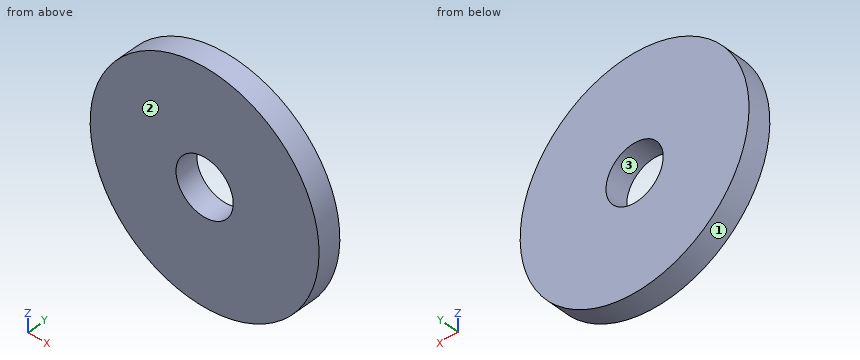
```python
from build123d import *

# Parameters (mm, degrees)
SKETCH1_R           = 12.5
SKETCH1_R_2         = 2.125
BOSS_EXTRUDE1_DEPTH = 2
SKETCH2_R           = 2.5
CUT_EXTRUDE1_DEPTH  = 10
CUT_EXTRUDE2_START  = -10
SKETCH3_R           = 12.5
SKETCH3_R_2         = 10
CUT_EXTRUDE2_DEPTH  = 10


with BuildPart() as part:
    # Sketch1 → Boss-Extrude1 (new body)
    with BuildSketch(Plane(origin=(0, 0, 0), x_dir=(1, 0, 0), z_dir=(0, 1, 0))):
        with Locations(Location((0, 0, 0), (0, 0, 270))):
            Circle(SKETCH1_R)
        with Locations(Location((0, 0, 0), (0, 0, 270))):
            Circle(SKETCH1_R_2, mode=Mode.SUBTRACT)
    extrude(amount=BOSS_EXTRUDE1_DEPTH)

    # Sketch2 → Cut-Extrude1 (cut)
    with BuildSketch(Plane(origin=(0, 2, 0), x_dir=(1, 0, 0), z_dir=(0, 1, 0))):
        with Locations(Location((0, 0, 0), (0, 0, 270))):
            Circle(SKETCH2_R)
    extrude(amount=-CUT_EXTRUDE1_DEPTH, mode=Mode.SUBTRACT)

    # Sketch3 → Cut-Extrude2 (cut)
    with BuildSketch(Plane(origin=(0, 2, 0), x_dir=(1, 0, 0), z_dir=(0, 1, 0)).offset(CUT_EXTRUDE2_START)):
        Circle(SKETCH3_R)
        with Locations(Location((0, 0, 0), (0, 0, 270))):
            Circle(SKETCH3_R_2, mode=Mode.SUBTRACT)
    extrude(amount=CUT_EXTRUDE2_DEPTH, mode=Mode.SUBTRACT)


solid = part.part
```
Verification items for the finished model (mm, model axes). Face numbers are marked on the shaded views. Give positions to 0.01 mm unless a question says otherwise; leave off trailing zeros. Order: outer loops, then holes, each group sorted by start corner. A loop starts at its lowest first (then second) coordinate and runs counter-clockwise, first axis right, second up. Notation, with made-up numbers: M 11.5,82.5 L 48.5,82.5 A3 ccw 48.5,87.5 Z; hole C -21,79.5 d1. An arc over 180 degrees is marked long. Return JSON: item names as keys, results as strings. Group by question number.
1) Scan lines: line 1 (X direction, y = 1.25, z = 0); line 2 (Z direction, x = -1.5, y = 1.6); line 3 (Z direction, x = 0.5, y = 0.25). Record each from-to range of solid material in increasing order.
2) Mould release check, pull along X, two halves, no side actions. Record for the marked faces 1, 2 and 3: pulls with the +X half, pulls with the -X half, needs draft (parallel to the pull), parting line crosses it, or undercut.
3) Section check C-C on y = 0.25. Record the cut outline in (x, z), and give its area (3 significant figures).
4) Section check A-A on z = 0. Record the cut outline in (x, y), and give its area (3 significant figures).
5) Section check D-D on z = 6.75. Record the cut outline in (x, y), and give its area (3 significant figures).
6) Section check B-B on x = 0. Record the cut outline in (y, z).
7) Go/stop test with flat-tipped pins: pin 1 Ø1 at (y, z) = (1, 1.5) entering from -X; pin 2 Ø4 at (x, z) = (0, 0) entering from +Y. Record where each tip stops, or that it passes through.
Answer block:
{
 "1": {"line 1": "x = -10 to -2.5, 2.5 to 10", "line 2": "z = -9.89 to -2, 2 to 9.89", "line 3": "z = -9.99 to -2.45, 2.45 to 9.99"},
 "2": {"face 1": "parting line crosses it", "face 2": "needs draft", "face 3": "undercut"},
 "3": {"outline": "C 0,0 d20; hole C 0,0 d5", "area": "295 mm^2"},
 "4": {"outline": "M -10,0 L -2.5,0 L -2.5,2 L -10,2 Z; M 2.5,0 L 10,0 L 10,2 L 2.5,2 Z", "area": "30.0 mm^2"},
 "5": {"outline": "M -7.38,0 L 7.38,0 L 7.38,2 L -7.38,2 Z", "area": "29.5 mm^2"},
 "6": {"outline": "M 0,-10 L 2,-10 L 2,-2.5 L 0,-2.5 Z; M 0,2.5 L 2,2.5 L 2,10 L 0,10 Z"},
 "7": {"pin 1": "stops at x = -9.95", "pin 2": "passes through"}
}
